The listing builds one solid part. Answer for the finished solid, in the listing's coordinates (mm). A direction names the side the tool comes from. Give positions to 0.01 mm unless a question says otherwise; leave off trailing zeros. Loops run counter-clockwise (first coordinate to the right, second up) from the corner with the lowest first, then second, coordinate; pieces in that order, holes last.
Item 1: The mould has two halves that part along X. Classify faces 1 (the face through (14, 8, 0)), 2 (the face through (4, 13, 0)), 3 (the face through (12.5, 4, 0)): pulls with the +X half, pulls with the -X half, needs draft (parallel to the pull), parting line crosses it, or undercut.
Item 2: Each of these flat-tipped pins is pushed along its axis until it touches: pin 1 Ø1.5 at (x, z) = (11, 0) entering from -Y; pin 2 Ø3 at (x, y) = (9.5, 9.5) entering from +Z; pin 3 Ø2.5 at (x, z) = (12.5, -0.5) entering from +Y; pin 4 Ø0.5 at (y, z) = (4.5, -2) entering from +X. Where does it stop, or does it pass through?
Item 3: Section A-A, the plane z = 2.5 is taken. Give the vertices of the cut face in (x, y), and give its area (3 significant figures).
Item 4: A tool of negligible diameter and unlimited length cuts with its end or side. For faces 4 (the face through (13, 5, 0)), 5 (the face through (5, 12.5, 0)), 6 (the face through (4.07, 9.79, -0.16)), from which of +Z, -Z, +X, -X, +Y, -Y can it reach the whole face along a straight path? Write none if from no direction.
Item 5: Consider line 1 along X through (y, z) = (9.5, 0.25); line 2 along Z through (x, y) = (6, 11). Determine where each line is inside the solid, lowest interval first.
Item 6: Section D-D, the plane x = 1 is taken. Give the vertices of the cut face in (y, z), and give its area (3 significant figures).
Item 7: Section B-B, the plane x = 9.5 is taken. Give the vertices of the cut face in (y, z).
Item 8: Section C-C, the plane z = 0 is taken. Give the vertices of the cut face in (x, y), and give its area (3 significant figures).
Autodesk Inventor part; units mm, degrees
ref_plane "YZ Plane" through (0, 0, 0) normal (1, 0, 0) x (0, 1, 0)
ref_plane "XZ Plane" through (0, 0, 0) normal (0, 1, 0) x (-1, 0, 0)
ref_plane "XY Plane" through (0, 0, 0) normal (0, 0, 1) x (1, 0, 0)
sketch "Sketch1" plane through (0, 0, 0) normal (0, 0, 1) x (1, 0, 0)
  line L0 (0, 0) -> (14, 0)
  line L1 (14, 0) -> (14, 14)
  line L2 (14, 14) -> (0, 14)
  line L3 (0, 14) -> (0, 0)
  dimension "d0" = 14
  dimension "d1" = 14
extrude "Extrusion1" add sketch "Sketch1" along normal mid plane 7
hole "Hole1" at (9.5, 9.5, 3.5) direction (0, 0, -1) diameter 4.7752 end through all
sketch "Sketch22" plane through (0, 0, 3.5) normal (0, 0, 1) x (1, 0, 0)
  line L0 (0, 0) -> (0, 14)
  line L1 (14, 0) -> (0, 0)
  arc A0 (8.5, 0) -> (0, 8.5) centre (0, 0) ccw
  line L2 (0, 8.5) -> (0, 0)
  line L3 (0, 0) -> (8.5, 0)
  dimension "d145" = 8.5
extrude "Extrusion19" cut sketch "Sketch22" against normal through all
sketch "Sketch15" plane through (0, 0, 3.5) normal (0, 0, 1) x (1, 0, 0)
  line L0 (14, 0) -> (0, 0)
  line L1 (0, 0) -> (0, 14)
  line L2 (5, 5) -> (5, 12)
  line L3 (5, 12) -> (4, 12)
  line L4 (4, 12) -> (4, 5)
  line L5 (5, 4) -> (12, 4)
  line L6 (12, 4) -> (12, 5)
  line L7 (12, 5) -> (5, 5)
  arc A0 (8.5, 0) -> (0, 8.5) centre (0, 0) ccw
  line L8 (4, 5) -> (0, 5)
  line L9 (0, 5) -> (0, 0)
  line L10 (0, 0) -> (5, 0)
  line L11 (5, 0) -> (5, 4)
  point P0 (0, 7.5)
  point P1 (7.5, 0)
  point P2 (5.3543, 6.6016)
  dimension "d94" = 1
  dimension "d95" = 4
  dimension "d96" = 4
  dimension "d97" = 12
extrude "sawblade" [suppressed]
chamfer "Chamfer5" distance 3 angle 45 1 edges at (14, 14, 0)
chamfer "Chamfer8" distance 0.5 angle 45 4 edges at (11.25, 0, 3.5) (0, 11.25, 3.5) (11.25, 0, -3.5) (0, 11.25, -3.5)
chamfer "Chamfer9" distance 0.5 angle 45 2 edges at (9.5, 11.8876, 3.5) (9.5, 11.8876, -3.5)
hole "Hole6" at (11, 0, 0) direction (0, 1, 0) diameter 2.4384 depth 8 tip angle 118 countersink diameter 2.54 countersink angle 120
hole "Hole7" at (0, 11, 0) direction (1, 0, 0) diameter 2.4384 depth 8 tip angle 118 countersink diameter 2.54 countersink angle 120
sketch "Sketch25" plane through (0, 0, 3.5) normal (0, 0, 1) x (1, 0, 0)
  line L0 (0.5, 14) -> (11, 14)
  line L1 (5, 14) -> (4, 14)
  line L2 (4, 14) -> (4, 11)
  line L3 (4, 11) -> (5, 11)
  line L4 (5, 11) -> (5, 14)
  line L5 (0, 14) -> (0, 8.5)
  dimension "d183" = 3
  dimension "d184" = 4
  dimension "d185" = 1
extrude "sawblade1" cut sketch "Sketch25" against normal through all
sketch "Sketch26" plane through (0, 0, 3.5) normal (0, 0, 1) x (1, 0, 0)
  line L0 (14, 5) -> (11, 5)
  line L1 (11, 5) -> (11, 4)
  line L2 (11, 4) -> (14, 4)
  line L3 (14, 4) -> (14, 5)
  line L4 (8.5, 0) -> (14, 0)
  dimension "d188" = 4
  dimension "d189" = 1
  dimension "d190" = 3
extrude "sawblade2" cut sketch "Sketch26" against normal through all
hole "Hole8" [suppressed]
hole "Hole9" [suppressed]
properties part number "FOX-ME-118-01" material "Delrin, Black"
Worked answers:
1. face 1: pulls with the +X half
1. face 2: undercut
1. face 3: needs draft
2. pin 1: stops at y = 8.28
2. pin 2: passes through
2. pin 3: stops at y = 13.75
2. pin 4: stops at x = 11
3. outline: (0, 8.5) arc R8.5 cw to (8.5, 0) - (14, 0) - (14, 4) - (11, 4) - (11, 5) - (14, 5) - (14, 11) - (11, 14) - (5, 14) - (5, 11) - (4, 11) - (4, 14) - (0, 14) - close; hole circle Ø4.78 at (9.5, 9.5)
3. area: 111 mm2
4. face 4: +Z, -Z, +X
4. face 5: +Z, -Z, +Y
4. face 6: -X
5. line 1: x = 0 to 7.11, 11.89 to 14
5. line 2: z = -3.5 to -1.22, 1.22 to 3.5
6. outline: (8.44, -3.5) - (14, -3.5) - (14, 3.5) - (8.44, 3.5) - close; hole circle Ø2.44 at (11, 0)
6. area: 34.2 mm2
7. outline: (0, -3) - (0.5, -3.5) - (6.61, -3.5) - (7.11, -3) - (7.11, 3) - (6.61, 3.5) - (0.5, 3.5) - (0, 3) - close; (11.89, -3) - (12.39, -3.5) - (14, -3.5) - (14, 3.5) - (12.39, 3.5) - (11.89, 3) - close
8. outline: (0, 8.5) arc R8.5 cw to (8.5, 0) - (9.73, 0) - (9.78, 0.03) - (9.78, 7.13) arc R2.39 cw to (7.13, 9.78) - (0.03, 9.78) - (0, 9.73) - close; (0, 12.27) - (0.03, 12.22) - (4, 12.22) - (4, 14) - (0, 14) - close; (5, 12.22) - (8, 12.22) - (8.37, 11.6) arc R2.39 cw to (11.6, 8.37) - (12.22, 8) - (12.22, 5) - (14, 5) - (14, 11) - (11, 14) - (5, 14) - close; (12.22, 0.03) - (12.27, 0) - (14, 0) - (14, 4) - (12.22, 4) - close
8. area: 75.8 mm2
